Model file for the job. Use its own axes, mm. A direction names the side the tool comes from. Give positions to 0.01 mm unless a question says otherwise; leave off trailing zeros. Loops run counter-clockwise (first coordinate to the right, second up) from the corner with the lowest first, then second, coordinate; pieces in that order, holes last. Notation, with made-up numbers: M -33,77 L 13,77 A18 ccw 13,104 Z; hole C 23,76 d1. An arc over 180 degrees is marked long. Answer in a Markdown table with one row per item.
```python
from build123d import *

# Parameters (mm, degrees)
F0_W     = 74
F0_H     = 74
F0_W_2   = 70
F0_H_2   = 70
F1_DEPTH = 10
F2_DEPTH = 2
F3_W     = 71.8
F3_H     = 71.8
F3_W_2   = 70
F3_H_2   = 70
F4_DEPTH = 2.7
F5_R     = 2


with BuildPart() as f1:
    # F0 (on Top) → F1 (new body)
    with BuildSketch(Plane.XY):
        with Locations((-2, -2)):
            Rectangle(F0_W, F0_H)
        with Locations((-2, -2)):
            Rectangle(F0_W_2, F0_H_2, mode=Mode.SUBTRACT)
    extrude(amount=F1_DEPTH)

    # F0 (on Top) → F2 (join)
    with BuildSketch(Plane.XY):
        with Locations((-2, -2)):
            Rectangle(F0_W_2, F0_H_2)
    extrude(amount=F2_DEPTH)

    # F3 (on face) → F4 (join)
    with BuildSketch(Plane.XY.offset(10)):
        with Locations((-2, -2)):
            Rectangle(F3_W, F3_H)
        with Locations((-2, -2)):
            Rectangle(F3_W_2, F3_H_2, mode=Mode.SUBTRACT)
    extrude(amount=F4_DEPTH)

    # F5
    f5_edges = [f1.edges().sort_by_distance(p)[0] for p in [
        (-39, -39, 5),
        (35, -39, 5),
        (35, 35, 5),
        (-39, 35, 5),
    ]]
    fillet(f5_edges, radius=F5_R)


solid = f1.part
```
(1) Saw through at B-B, the plane y = -3.5. Give the cut face in (x, z).
Established:
| item | result |
|---|---|
| outline | M -39,0 L 35,0 L 35,10 L 33.9,10 L 33.9,12.7 L 33,12.7 L 33,2 L -37,2 L -37,12.7 L -37.9,12.7 L -37.9,10 L -39,10 Z |
(2) Which spindle directions (+Z, -Z, +X, -X, +Y, -Y) get a long thin tool onto all of the face, cutting with end or side? Do faces 5 (the flat face through (-2, -2, 2)), 6 (the flat face through (-2, -39, 5)), 7 (the flat face through (33.9, -3, 11)), 8 (the flat face through (-3, 33.9, 11)), 9 (the cylindrical face through (-38.4, 34.43, 5.07)). Say none if no direction does.
Established:
| item | result |
|---|---|
| face 5 | +Z |
| face 6 | +Z, -Z, +X, -X, -Y |
| face 7 | +Z, +X, +Y, -Y |
| face 8 | +Z, +X, -X, +Y |
| face 9 | +Z, -Z, -X, +Y |
(3) Mould opens along X. For faces 1 (the cylindrical face through (34.43, -38.4, 5.07)), 2 (the flat face through (-2, 33, 7)), 3 (the flat face through (-2, -37, 7)), 4 (the flat face through (-3, -37.9, 11)) say: pulls with the +X half, pulls with the -X half, needs draft (parallel to the pull), parting line crosses it, or undercut.
Established:
| item | result |
|---|---|
| face 1 | pulls with the +X half |
| face 2 | undercut |
| face 3 | undercut |
| face 4 | needs draft |
(4) Flat gauge pins, fed straight in: P1, Ø10, axis at x = -10, y = -31.5, coming from the -Z side; P2, Ø0.8, axis at x = -11.5, z = 11, coming from the +Y side; P3, Ø1.3, axis at x = 13.5, z = 11.5, coming from the -Y side; P4, Ø2, axis at x = 9, y = 1, coming from the +Z side. Where does each tip first touch, or does it go through?
Established:
| item | result |
|---|---|
| P1 | stops at z = 0 |
| P2 | stops at y = 33.9 |
| P3 | stops at y = -37.9 |
| P4 | stops at z = 2 |
(5) Saw through at A-A, the plane z = 7. Give the cut face in (x, y), and give its area (3 significant figures).
Established:
| item | result |
|---|---|
| outline | M -39,-37 A2 ccw -37,-39 L 33,-39 A2 ccw 35,-37 L 35,33 A2 ccw 33,35 L -37,35 A2 ccw -39,33 Z; hole M -37,-37 L 33,-37 L 33,33 L -37,33 Z |
| area | 573 mm2 |
(6) Wall check: L1, parallel to X at y = -12, z = 11; L2, parallel to X at y = 14, z = 3. Give the ranges that are in metal, low to high.
Established:
| item | result |
|---|---|
| L1 | x = -37.9 to -37, 33 to 33.9 |
| L2 | x = -39 to -37, 33 to 35 |
